Geometry: final body of the model. Coordinates: model frame, mm. A direction names the side the tool comes from. Coordinates: 2 decimals unless noted, no trailing zeros. Order: outer loops, then holes, each group sorted by start corner. A loop starts at its lowest first (then second) coordinate and runs counter-clockwise, first axis right, second up. Notation, with made-up numbers: (33, -2) -> (73, -2) arc R23 ccw to (73, 24) -> close; hole circle Ø11 at (29.5, 1). An arc over 180 degrees is marked (long way). Answer in a Markdown table with one row per item. Add a question column.
1) Section query B-B on z = 0. Return the cut outline in (x, y).
2) Section query A-A on y = -3.75. Return the cut outline in (x, z).
3) Pull-direction query (X, two-part tool) for faces 1 (the face through (20, -4, 0)), 2 (the face through (-17.15, -3.94, -16.99)), 3 (the face through (12.208, -7.014, -3.644)); classes: +X half, -X half, draft (parallel to the pull), parting line (faces both ways), or undercut.
4) Ray query, line 1 (Z direction, x = 0, y = -6.95); line 2 (Y direction, x = 9, z = 2.5); line 3 (Y direction, x = 11.5, z = -6.5). Return the intervals inside material, ascending. Write a range as from..to.
5) Section query D-D on y = -8.75. Return the cut outline in (x, z).
6) Section query C-C on x = 0. Return the cut outline in (y, z), then the cut area to 3 significant figures.
7) Set-up query: faces 4 (the face through (-16, -10, 0)), 5 (the face through (-4.58, -7.01, -3.64)). Return all of +Z, -Z, +X, -X, +Y, -Y with unobstructed straight access to the full face (end or side cutting, diameter ignored); none if empty.
8) Contact query for flat-ended pins moving along their axis: P1, Ø4, axis at x = 1.5, z = 9.5, coming from the -Y side; P2, Ø6.5, axis at x = 8.5, z = -6.5, coming from the -Y side; P3, Ø3, axis at y = -5.5, z = 12.5, coming from the -X side. Output: stop coordinate, or through.
```python
from build123d import *

# Parameters (mm, degrees)
F0_W         = 40
F0_H         = 40
F1_DEPTH     = 10
F2_R         = 15.5
F3_DEPTH     = 2
F4_R         = 4
F5_DEPTH     = 2
F6_R         = 2
F7_T1_DEPTH  = 35
F7_T4_ANGLE  = 90
F7_T6_ANGLE  = 90
F7_T8_ANGLE  = 90
F7_T10_ANGLE = 90


# Not quite as in the source:
# - a fillet or chamfer that OpenCascade refuses, or shapes differently, is made with other operations: its cross-section is extruded or revolved along the edge and cut away or added


with BuildPart() as f1:
    # F0 (on Front) → F1 (new body)
    with BuildSketch(Plane.XZ):
        Rectangle(F0_W, F0_H)
    extrude(amount=F1_DEPTH)

    # F2 (on face) → F3 (cut)
    with BuildSketch(Plane.XZ.offset(10)):
        Circle(F2_R)
    extrude(amount=-F3_DEPTH, mode=Mode.SUBTRACT)

    # F4 (on face) → F5 (cut)
    with BuildSketch(Plane.XZ.offset(8)):
        with Locations((0, 9.6908602864)):
            Circle(F4_R)
        with Locations((-8.3925311925, -4.8454301432)):
            Circle(F4_R)
        with Locations((8.3925311925, -4.8454301432)):
            Circle(F4_R)
    extrude(amount=-F5_DEPTH, mode=Mode.SUBTRACT)

    # F6
    f6_edges = [f1.edges().sort_by_distance(p)[0] for p in [
        (0, -10, 20),
        (-20, -10, 0),
        (20, -10, 0),
        (0, -10, -20),
    ]]
    fillet(f6_edges, radius=F6_R)

    # F7: fillet of radius 10 on 4 edges, made by hand

    # F7_s2 → F7_t1 (cut)
    with BuildSketch(Plane.XZ.offset(-25)):
        with BuildLine():
            ThreePointArc((10, 20), (17.0710678119, 17.0710678119), (20, 10))
            Line((20, 10), (20, 20))
            Line((20, 20), (10, 20))
        make_face()
        with BuildLine():
            ThreePointArc((-10, 20), (-17.0710678119, 17.0710678119), (-20, 10))
            Line((-20, 10), (-20, 20))
            Line((-20, 20), (-10, 20))
        make_face()
        with BuildLine():
            ThreePointArc((20, -10), (17.0710678119, -17.0710678119), (10, -20))
            Line((10, -20), (20, -20))
            Line((20, -20), (20, -10))
        make_face()
        with BuildLine():
            ThreePointArc((-20, -10), (-17.0710678119, -17.0710678119), (-10, -20))
            Line((-10, -20), (-20, -20))
            Line((-20, -20), (-20, -10))
        make_face()
    extrude(amount=F7_T1_DEPTH, mode=Mode.SUBTRACT)

    # F7_s3 → F7_t4 (revolve, cut)
    with BuildSketch(Plane.XY.offset(-10)):
        with BuildLine():
            ThreePointArc((-18, -10), (-19.4142135624, -9.4142135624), (-20, -8))
            Line((-20, -8), (-20, -10))
            Line((-20, -10), (-18, -10))
        make_face()
    revolve(axis=Axis((-10, -10, -10), (0, -1, 0)), revolution_arc=F7_T4_ANGLE, mode=Mode.SUBTRACT)

    # F7_s5 → F7_t6 (revolve, cut)
    with BuildSketch(Plane.YZ.offset(10)):
        with BuildLine():
            ThreePointArc((-10, -18), (-9.4142135624, -19.4142135624), (-8, -20))
            Line((-8, -20), (-10, -20))
            Line((-10, -20), (-10, -18))
        make_face()
    revolve(axis=Axis((10, -10, -10), (0, -1, 0)), revolution_arc=F7_T6_ANGLE, mode=Mode.SUBTRACT)

    # F7_s7 → F7_t8 (revolve, cut)
    with BuildSketch(Plane.YZ.offset(-10)):
        with BuildLine():
            ThreePointArc((-10, 18), (-9.4142135624, 19.4142135624), (-8, 20))
            Line((-8, 20), (-10, 20))
            Line((-10, 20), (-10, 18))
        make_face()
    revolve(axis=Axis((-10, -10, 10), (0, -1, 0)), revolution_arc=F7_T8_ANGLE, mode=Mode.SUBTRACT)

    # F7_s9 → F7_t10 (revolve, cut)
    with BuildSketch(Plane.XY.offset(10)):
        with BuildLine():
            ThreePointArc((18, -10), (19.4142135624, -9.4142135624), (20, -8))
            Line((20, -8), (20, -10))
            Line((20, -10), (18, -10))
        make_face()
    revolve(axis=Axis((10, -10, 10), (0, -1, 0)), revolution_arc=F7_T10_ANGLE, mode=Mode.SUBTRACT)


solid = f1.part
```
Result:
| question | item | result |
|---|---|---|
| 1 | outline | (-20, -8) arc R2 ccw to (-18, -10) -> (-15.5, -10) -> (-15.5, -8) -> (15.5, -8) -> (15.5, -10) -> (18, -10) arc R2 ccw to (20, -8) -> (20, 0) -> (-20, 0) -> close |
| 2 | outline | (-20, -10) arc R10 ccw to (-10, -20) -> (10, -20) arc R10 ccw to (20, -10) -> (20, 10) arc R10 ccw to (10, 20) -> (-10, 20) arc R10 ccw to (-20, 10) -> close |
| 3 | face 1 | +X half |
| 3 | face 2 | -X half |
| 3 | face 3 | undercut |
| 4 | line 1 | -20..5.69, 13.69..20 |
| 4 | line 2 | -8..0 |
| 4 | line 3 | -6..0 |
| 5 | outline | (-19.85, -10) arc R9.85 ccw to (-10, -19.85) -> (10, -19.85) arc R9.85 ccw to (19.85, -10) -> (19.85, 10) arc R9.85 ccw to (10, 19.85) -> (-10, 19.85) arc R9.85 ccw to (-19.85, 10) -> close; hole circle Ø31 at (0, 0) |
| 6 | outline | (-10, -18) arc R2 ccw to (-8, -20) -> (0, -20) -> (0, 20) -> (-8, 20) arc R2 ccw to (-10, 18) -> (-10, 15.5) -> (-8, 15.5) -> (-8, 13.69) -> (-6, 13.69) -> (-6, 5.69) -> (-8, 5.69) -> (-8, -15.5) -> (-10, -15.5) -> close |
| 6 | area | 320 mm2 |
| 7 | face 4 | +Z, -Z, +X, -X, -Y |
| 7 | face 5 | -Y |
| 8 | P1 | y = -6 |
| 8 | P2 | y = -8 |
| 8 | P3 | x = -19.95 |
